```python
from build123d import *

# Parameters (mm, degrees)
SKETCH1_W   = 15.875
SKETCH1_H   = 12.7
SKETCH8_W   = 22.5425
SKETCH8_H   = 11
SKETCH8_W_2 = 2.8575
SKETCH8_H_2 = 7.62


with BuildPart() as part:
    # Sketch1 → Colar press section (revolve)
    with BuildSketch(Plane.XY, mode=Mode.PRIVATE) as colar_press_section_sk:
        with Locations((0, 6.35)):
            Rectangle(SKETCH1_W, SKETCH1_H)
    revolve(colar_press_section_sk.sketch.rotate(Axis((-7.9375, 0, 0), (1, 0, 0)), 90), axis=Axis((-7.9375, 0, 0), (1, 0, 0)))

    # Sketch7 → Revolve2 (revolve)
    with BuildSketch(Plane.XY):
        with BuildLine():
            Line((12.7, -0.762), (7.9375, -0.762))
            Line((7.9375, -0.762), (7.9375, 15.24))
            Line((7.9375, 15.24), (9.128125, 15.24))
            ThreePointArc((9.128125, 15.24), (10.31875, 14.049375), (11.509375, 15.24))
            Line((11.509375, 15.24), (12.7, 15.24))
            Line((12.7, 15.24), (12.7, -0.762))
        make_face()
        Polygon((-12.7, -0.762), (-7.9375, -0.762), (-7.9375, -12.7), (-9.128125, -12.7), (-11.509375, -12.7), (-12.7, -12.7), align=None)
    revolve(axis=Axis((39.064984039, -0.762, 0), (-1, 0, 0)))

    # Sketch8 → Cut-Revolve3 (revolve, cut)
    with BuildSketch(Plane.XY):
        with Locations((-1.42875, 4.738)):
            Rectangle(SKETCH8_W, SKETCH8_H)
        with Locations((11.27125, 3.048)):
            Rectangle(SKETCH8_W_2, SKETCH8_H_2)
    revolve(axis=Axis((39.064984039, -0.762, 0), (-1, 0, 0)), mode=Mode.SUBTRACT)


solid = part.part
```
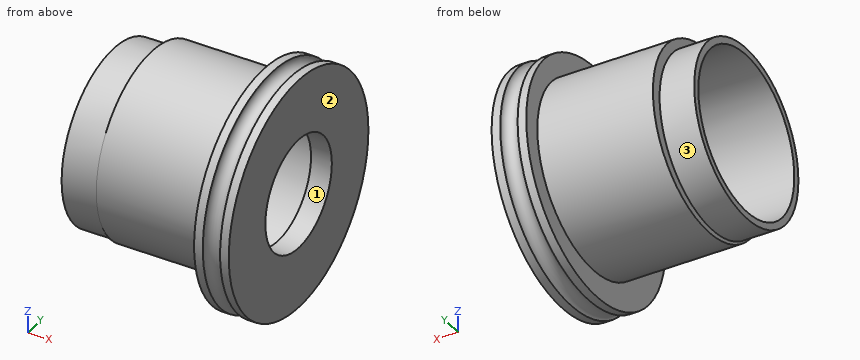
Model file for the job. Use its own axes, mm. Face numbers are marked on the shaded views. Round coordinates to 2 decimals unless told otherwise and drop trailing zeros. Loops run counter-clockwise (first coordinate to the right, second up) from the corner with the lowest first, then second, coordinate; pieces in that order, holes last. Notation, with made-up numbers: M 47,77 L 99,77 A18 ccw 99,87 Z; hole C 70,-10 d5. An arc over 180 degrees is marked long. Put each result on its own line as item: value. Start each with the question number.
Item 1: Cut at A-A (x = 7.5). List the corners of the cut face in (y, z), then the cut area to 3 significant figures.
Item 2: Drill centre lines: line 1 along Z through (x, y) = (6.75, -0.5); line 2 along Y through (x, z) = (4.5, 0); line 3 along Y through (x, z) = (12.05, 0). Where is each one in solid material? Low to high.
Item 3: Drop flat-ended pins along their axis: P1, Ø5, axis at x = -0.5, z = -11.5, coming from the +Y side; P2, Ø10, axis at x = 0.5, y = -10.5, coming from the +Z side; P3, Ø12, axis at x = -9, z = -7.5, coming from the +Y side. Give the stop position or say it passes through.
Item 4: Mould opens along Z. For the marked faces 1, 2 and 3 say: released by +Z, released by -Z, zero draft, split by the parting line, or undercut.
Answer block:
1. outline: C 0,0 d25.4; hole C -0.76,0 d22
1. area: 127 mm2
2. line 1: -12.69 to -11, 11 to 12.69
2. line 2: -12.7 to -11.76, 10.24 to 12.7
2. line 3: -16.76 to -8.38, 6.86 to 15.24
3. P1: y = 8.96
3. P2: z = 11.45
3. P3: y = 12.6
4. face 1: undercut
4. face 2: zero draft
4. face 3: split by the parting line
